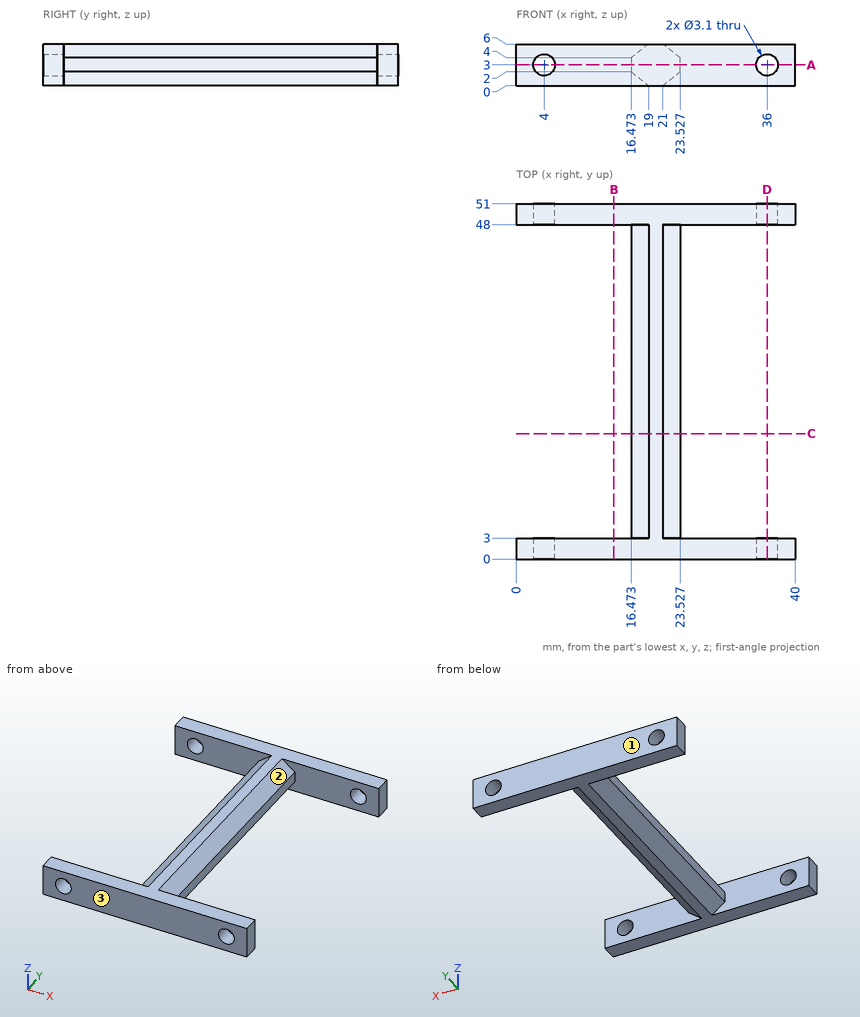
Geometry check sheet. Reference: drawing and pictorial views, mm from the part's lowest x, y, z. Coordinates: 2 decimals unless noted, no trailing zeros. Write each loop counter-clockwise with the first axis right and the second up, starting at its lowest first coordinate (ties: lowest second). Pieces come first, ordered by that corner, then holes. Notation, with made-up numbers: M 9.25,-24 L 18.25,-24 A18 cw 18.25,-7 Z; hole C 22.25,18.25 d9. An arc over 180 degrees is marked long. One line per question, with ' | ' between items.
1) Sectioned sample at C-C on y = 18. Record the cut outline in (x, z), then the cut area to 3 significant figures.
Solutions:
outline: M 16.47,2 L 19,0 L 21,0 L 23.53,2 L 23.53,4 L 21,6 L 19,6 L 16.47,4 Z | area: 32.2 mm^2
2) Sectioned sample at B-B on x = 14. Record the cut outline in (y, z).
Solutions:
outline: M 0,0 L 3,0 L 3,6 L 0,6 Z; M 48,0 L 51,0 L 51,6 L 48,6 Z
3) Sectioned sample at D-D on x = 36. Record the cut outline in (y, z), then the cut area to 3 significant figures.
Solutions:
outline: M 0,0 L 3,0 L 3,1.45 L 0,1.45 Z; M 0,4.55 L 3,4.55 L 3,6 L 0,6 Z; M 48,0 L 51,0 L 51,1.45 L 48,1.45 Z; M 48,4.55 L 51,4.55 L 51,6 L 48,6 Z | area: 17.4 mm^2
4) Release check for a two-part mould opening along Y. For the marked faces 1, 2 and 3 record: +Y half, -Y half, draft (parallel to the pull), parting line (faces both ways), or undercut.
Solutions:
face 1: +Y half | face 2: undercut | face 3: -Y half
5) Sectioned sample at A-A on z = 3. Record the cut outline in (x, y), then the cut area to 3 significant figures.
Solutions:
outline: M 0,0 L 2.45,0 L 2.45,3 L 0,3 Z; M 0,48 L 2.45,48 L 2.45,51 L 0,51 Z; M 5.55,0 L 34.45,0 L 34.45,3 L 23.53,3 L 23.53,48 L 34.45,48 L 34.45,51 L 5.55,51 L 5.55,48 L 16.47,48 L 16.47,3 L 5.55,3 Z; M 37.55,0 L 40,0 L 40,3 L 37.55,3 Z; M 37.55,48 L 40,48 L 40,51 L 37.55,51 Z | area: 520 mm^2
6) Depth check by flat-ended pin: pin 1 Ø1.6 at (y, z) = (31.5, 2.5) entering from +X; pin 2 Ø2 at (y, z) = (16.5, 3) entering from -X. Enter the tip coordinate at first touch or a pass-through.
Solutions:
pin 1: x = 23.53 | pin 2: x = 16.47
7) Material ranges on L1, parallel to Y at x = 30, z = 4.35; L2, parallel to Z at x = 36, y = 49; L3, parallel to X at y = 6, z = 2.85, recorded low to high.
Solutions:
L1: 0 to 3, 48 to 51 | L2: 0 to 1.45, 4.55 to 6 | L3: 16.47 to 23.53
